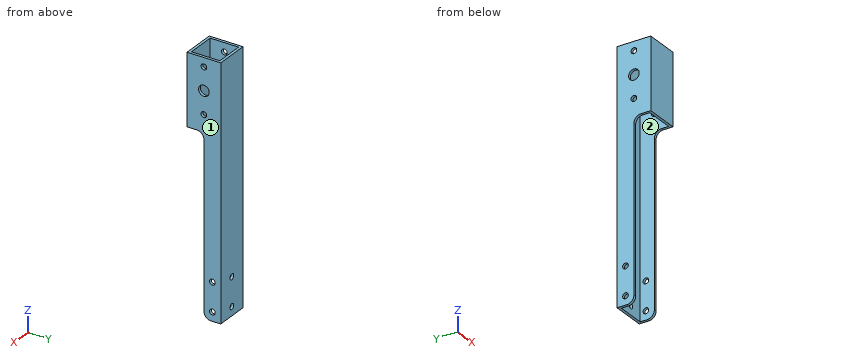
from build123d import *

# Parameters (mm, degrees)
ESBO_O1_W                = 19
ESBO_O1_H                = 19
ESBO_O1_W_2              = 16
ESBO_O1_H_2              = 16
RESSALTO_EXTRUS_O1_DEPTH = 140
ESBO_O2_R                = 1.6
ESBO_O2_R_2              = 3
CORTE_EXTRUS_O1_DEPTH    = 20
ESBO_O3_R                = 1.6
CORTE_EXTRUS_O2_DEPTH    = 1.5
ESBO_O5_W                = 19
ESBO_O5_H                = 9.5
CORTE_EXTRUS_O4_DEPTH    = 100
FILETE1_R                = 4


with BuildPart() as part:
    # Esboço1 → Ressalto-extrusão1 (new body)
    with BuildSketch(Plane.XY):
        Rectangle(ESBO_O1_W, ESBO_O1_H)
        Rectangle(ESBO_O1_W_2, ESBO_O1_H_2, mode=Mode.SUBTRACT)
    extrude(amount=RESSALTO_EXTRUS_O1_DEPTH)

    # Esboço2 → Corte-extrusão1 (cut, through all)
    with BuildSketch(Plane(origin=(9.5, 0, 0), x_dir=(0, 0, -1), z_dir=(1, 0, 0))):
        with Locations((-109.38750305, 0)):
            Circle(ESBO_O2_R)
        with Locations((-135, 0)):
            Circle(ESBO_O2_R)
        with Locations((-122.193751525, 0)):
            Circle(ESBO_O2_R_2)
        with Locations((-5, 4.75)):
            Circle(ESBO_O2_R)
        with Locations((-21, 4.75)):
            Circle(ESBO_O2_R)
    extrude(amount=-CORTE_EXTRUS_O1_DEPTH, mode=Mode.SUBTRACT)

    # Esboço3 → Corte-extrusão2 (cut)
    with BuildSketch(Plane(origin=(0, 9.5, 0), x_dir=(1, 0, 0), z_dir=(0, 1, 0))):
        with Locations((0, -21)):
            Circle(ESBO_O3_R)
        with Locations((0, -5)):
            Circle(ESBO_O3_R)
    extrude(amount=-CORTE_EXTRUS_O2_DEPTH, mode=Mode.SUBTRACT)

    # Esboço5 → Corte-extrusão4 (cut)
    with BuildSketch(Plane(origin=(0, 0, 0), x_dir=(-1, 0, 0), z_dir=(0, 0, -1))):
        with Locations((0, -4.75)):
            Rectangle(ESBO_O5_W, ESBO_O5_H)
    extrude(amount=-CORTE_EXTRUS_O4_DEPTH, mode=Mode.SUBTRACT)

    # Filete1
    filete1_edges = [part.edges().sort_by_distance(p)[0] for p in [
        (-8.75, 0, 0),
        (8.75, 0, 0),
        (-8.75, 0, 100),
        (8.75, 0, 100),
    ]]
    fillet(filete1_edges, radius=FILETE1_R)


solid = part.part
Read the model definition and answer for the solid it produces. Units are mm, in the model's axes. Face numbers are marked on the shaded views. A direction names the side the tool comes from. Round coordinates to 2 decimals unless told otherwise and drop trailing zeros. Write each loop counter-clockwise with the first axis right and the second up, starting at its lowest first coordinate (ties: lowest second). Pieces come first, ordered by that corner, then holes.
1. The part is cut by section A-A, the plane z = 21. Determine the outline of the cut face in (x, y).
2. The part is cut by section C-C, the plane x = 0. Determine the outline of the cut face in (y, z).
3. The part is cut by section B-B, the plane x = -6.75. Determine the outline of the cut face in (y, z).
4. The part is cut by section D-D, the plane z = 135. Determine the outline of the cut face in (x, y).
5. Straight lines are drawn through the part: L1, parallel to Z at x = 0, y = 9.2; L2, parallel to X at y = -1, z = 101; L3, parallel to Y at x = -8.35, z = 21. For each, find the intervals that lie inside material, in ascending order.
6. Given pin 1 Ø1.5 at (x, y) = (-3.5, -6) entering from -Z; pin 2 Ø8 at (x, y) = (2, -5) entering from -Z; pin 3 Ø8 at (x, y) = (7.5, -6) entering from -Z; pin 4 Ø1.6 at (x, z) = (9, 62) entering from -Y, each flat-ended and moving along its own axis, determine where each tip first touches the part or whether it passes through.
7. Which of the six approach directions +Z, -Z, +X, -X, +Y, -Y give full straight-line access (tool end or side, diameter ignored) to the marked faces 1 and 2?
Values:
1. outline: (-9.5, 0) - (-8, 0) - (-8, 3.15) - (-9.5, 3.15) - close; (-9.5, 6.35) - (-8, 6.35) - (-8, 8) - (-1.6, 8) - (-1.6, 9.5) - (-9.5, 9.5) - close; (1.6, 8) - (8, 8) - (8, 6.35) - (9.5, 6.35) - (9.5, 9.5) - (1.6, 9.5) - close; (8, 0) - (9.5, 0) - (9.5, 3.15) - (8, 3.15) - close
2. outline: (-9.5, 100) - (-8, 100) - (-8, 140) - (-9.5, 140) - close; (8, 0) - (9.5, 0) - (9.5, 3.4) - (8, 3.4) - close; (8, 6.6) - (9.5, 6.6) - (9.5, 19.4) - (8, 19.4) - close; (8, 22.6) - (9.5, 22.6) - (9.5, 140) - (8, 140) - close
3. outline: (-9.5, 100) - (-8, 100) - (-8, 140) - (-9.5, 140) - close; (8, 0) - (9.5, 0) - (9.5, 140) - (8, 140) - close
4. outline: (-9.5, -9.5) - (9.5, -9.5) - (9.5, -1.6) - (8, -1.6) - (8, -8) - (-8, -8) - (-8, -1.6) - (-9.5, -1.6) - close; (-9.5, 1.6) - (-8, 1.6) - (-8, 8) - (8, 8) - (8, 1.6) - (9.5, 1.6) - (9.5, 9.5) - (-9.5, 9.5) - close
5. L1: z = 0 to 3.4, 6.6 to 19.4, 22.6 to 140
5. L2: x = -9.5 to -8, 8 to 9.5
5. L3: y = 0 to 3.15, 6.35 to 9.5
6. pin 1: passes through
6. pin 2: stops at z = 100
6. pin 3: stops at z = 99.48
6. pin 4: stops at y = 0
7. face 1: +Z, -Z, +X, +Y, -Y
7. face 2: +Z, -Z
